Source: three-view drawing plus pictorial views. Frame: mm from the lowest corner of the part. Give positions to 0.01 mm unless a question says otherwise; leave off trailing zeros. Write each loop counter-clockwise with the first axis right and the second up, starting at its lowest first coordinate (ties: lowest second). Pieces come first, ordered by that corner, then holes. Notation, with made-up numbers: (9.5, 18.5) -> (45.5, 18.5) arc R8 ccw to (45.5, 30.5) -> close; hole circle Ø9 at (23.5, 70.5). An arc over 180 degrees is marked (long way). Use a Markdown table: item, result. Add a question column.
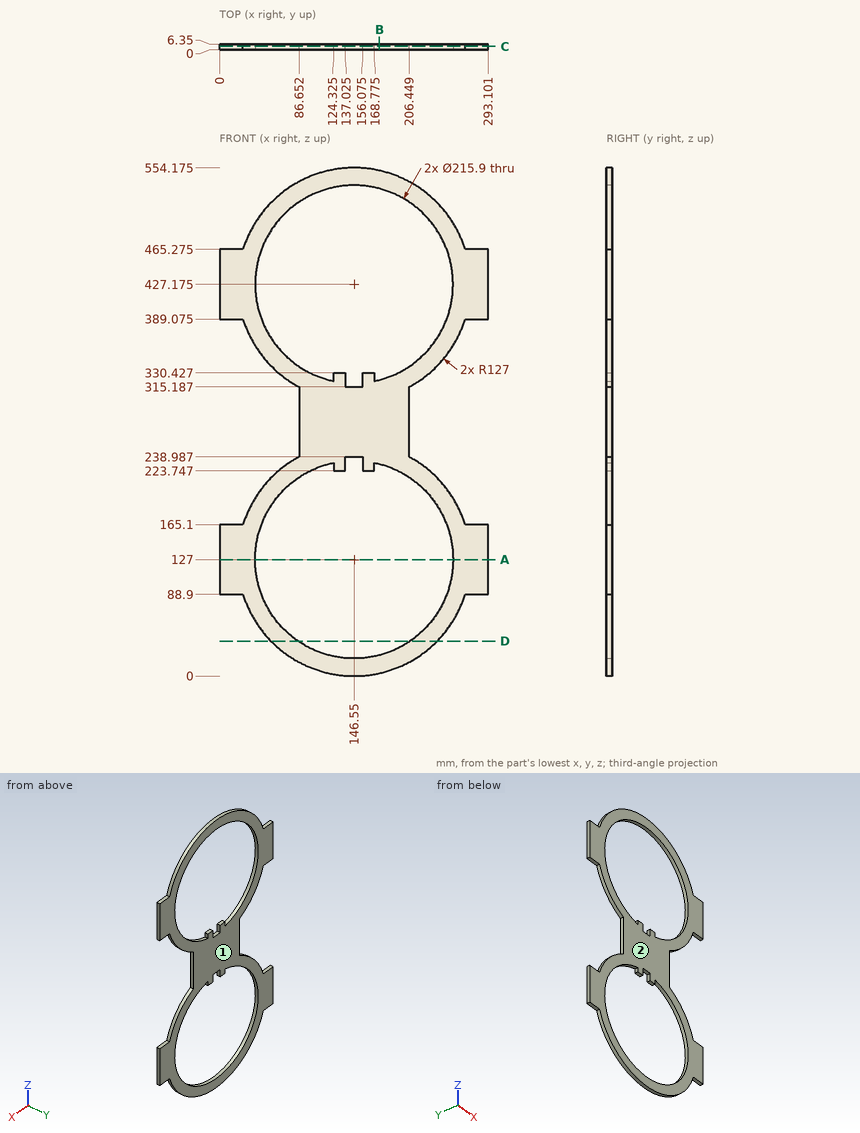
(1) Material intervals for L1, parallel to X at y = 4.75, z = 127; L2, parallel to Z at x = 19.5, y = 3 (1 decimal); L3, parallel to Z at x = 56.5, y = 5.5 (1 decimal), sorted ascending.
(2) First-contact query: pin 1 Ø3 at (y, z) = (2, 233.5) entering from +X; pin 2 Ø1.9 at (x, y) = (284.5, 1.5) entering from -Z; pin 3 Ø1.9 at (y, z) = (2, 287.5) entering from -X; pin 4 Ø8 at (x, z) = (251, 104) entering from -Y. Flat tips, straight axial feed; report the tip coordinate or a pass-through.
(3) Mould query, pull axis Y, two halves, no side actions, for the marked faces 1 and 2. Classes: +Y half, -Y half, draft (parallel to the pull), parting line (faces both ways), or undercut.
(4) Cut plane D-D on z = 38. Return the cut outline in (x, y).
(5) Cut plane B-B on x = 174. Return the cut outline in (y, z), then the cut area to 3 significant figures.
(6) Cut plane C-C on y = 3.75. Count the separate pieces of the cut face and the enclosed holes in it, then the cut area to 3 significant figures.
(7) Cut plane A-A on z = 127. Return the cut outline in (x, y), then the cut area to 3 significant figures.
Output:
| question | item | result |
|---|---|---|
| 1 | L1 | 0 to 38.6, 254.5 to 293.1 |
| 1 | L2 | 88.9 to 165.1, 389.1 to 465.3 |
| 1 | L3 | 37.4 to 67.5, 186.5 to 216.6, 337.6 to 367.6, 486.7 to 516.7 |
| 2 | pin 1 | x = 217.99 |
| 2 | pin 2 | z = 88.9 |
| 2 | pin 3 | x = 86.65 |
| 2 | pin 4 | y = 0 |
| 3 | face 1 | +Y half |
| 3 | face 2 | -Y half |
| 4 | outline | (55.95, 0) -> (85.46, 0) -> (85.46, 6.35) -> (55.95, 6.35) -> close; (207.64, 0) -> (237.15, 0) -> (237.15, 6.35) -> (207.64, 6.35) -> close |
| 5 | outline | (0, 3) -> (6.35, 3) -> (6.35, 22.6) -> (0, 22.6) -> close; (0, 231.4) -> (6.35, 231.4) -> (6.35, 322.77) -> (0, 322.77) -> close; (0, 531.58) -> (6.35, 531.58) -> (6.35, 551.17) -> (0, 551.17) -> close |
| 5 | area | 829 mm^2 |
| 6 | separate pieces | 1 |
| 6 | enclosed holes | 2 |
| 6 | area | 41,700 mm^2 |
| 7 | outline | (0, 0) -> (38.6, 0) -> (38.6, 6.35) -> (0, 6.35) -> close; (254.5, 0) -> (293.1, 0) -> (293.1, 6.35) -> (254.5, 6.35) -> close |
| 7 | area | 490 mm^2 |
